Can you work these out from the model? Positions are in its coordinate system, mm. Face numbers are marked on the shaded views. A direction names the side the tool comes from. Coordinates: 2 decimals unless noted, no trailing zeros. Loops run counter-clockwise (first coordinate to the right, second up) from the corner with the lowest first, then second, coordinate; pieces in that order, holes last.
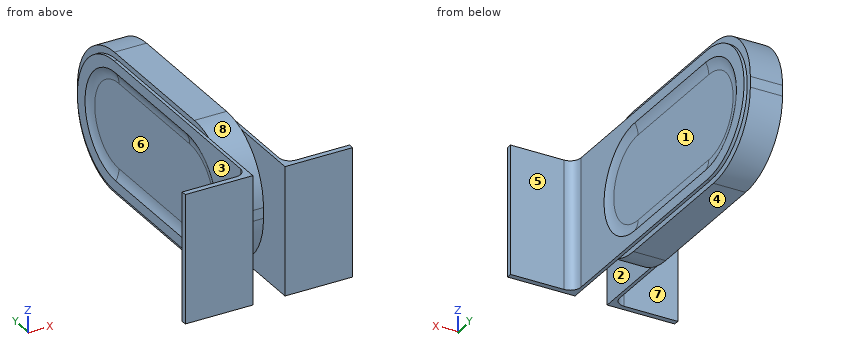
```python
from build123d import *

# Parameters (mm, degrees)
BOSS_EXTRUDE1_DEPTH = 15
BOSS_EXTRUDE2_DEPTH = 3
FILLET1_R           = 20
SKETCH4_W           = 60
SKETCH4_H           = 120
BOSS_EXTRUDE3_DEPTH = 5
BOSS_EXTRUDE4_START = -30
BOSS_EXTRUDE4_DEPTH = 3
FILLET2_R           = 20
FILLET4_R           = 10
BOSS_EXTRUDE5_START = -5
BOSS_EXTRUDE5_DEPTH = 120


with BuildPart() as part:
    # Sketch1 → Boss-Extrude1 (new, symmetric)
    with BuildSketch(Plane(origin=(0, 0, 0), x_dir=(0, 0, -1), z_dir=(1, 0, 0))):
        with BuildLine():
            Line((5, 125), (-5, 125))
            ThreePointArc((-5, 125), (-47.426406871, 107.426406871), (-65, 65))
            Line((-65, 65), (-65, -65))
            ThreePointArc((-65, -65), (-47.426406871, -107.426406871), (-5, -125))
            Line((-5, -125), (5, -125))
            ThreePointArc((5, -125), (47.426406871, -107.426406871), (65, -65))
            Line((65, -65), (65, 65))
            ThreePointArc((65, 65), (47.426406871, 107.426406871), (5, 125))
        make_face()
    extrude(amount=BOSS_EXTRUDE1_DEPTH, both=True)

    # Sketch3 → Boss-Extrude2 (add)
    with BuildSketch(Plane(origin=(15, 0, 0), x_dir=(0, 0, -1), z_dir=(1, 0, 0))):
        with BuildLine():
            Line((-60, -60), (-60, 60))
            ThreePointArc((-60, 60), (0, 120), (60, 60))
            Line((60, 60), (60, -60))
            Line((60, -60), (60, -160))
            Line((60, -160), (-60, -160))
            Line((-60, -160), (-60, -60))
        make_face()
        with BuildLine():
            Line((-50, -57.5), (-50, 57.5))
            ThreePointArc((-50, 57.5), (0, 107.5), (50, 57.5))
            Line((50, 57.5), (50, -57.5))
            ThreePointArc((50, -57.5), (0, -107.5), (-50, -57.5))
        make_face(mode=Mode.SUBTRACT)
    extrude(amount=BOSS_EXTRUDE2_DEPTH)

    # Fillet1
    # the kernel refuses this fillet: 20 mm, written as the material it adds along each edge
    with BuildSketch(Plane(origin=(15, 57.5, -50), x_dir=(1, 0, 0), z_dir=(0, -1, 0)), Plane(origin=(15, -57.5, 50), x_dir=(1, 0, 0), z_dir=(0, 1, 0))) as fillet1_piece_1:
        with BuildLine():
            CenterArc((20, 10.535653753), FILLET1_R, 180, 31.788330617)
            Line((0, 10.535653753), (-0.4, 10.535653753))
            Line((-0.4, 10.535653753), (-0.4, 0))
            Line((-0.4, 0), (0, -0.4))
            ThreePointArc((0, -0.4), (1.5, -0.4), (2.66, -0.210713075))
            Line((2.66, -0.210713075), (3, 0))
        make_face()
    extrude(amount=115)
    with BuildSketch(Plane(origin=(15, -57.5, 0), x_dir=(0, 0, -1), z_dir=(0, 1, 0))) as fillet1_piece_2:
        with BuildLine():
            CenterArc((39.464346247, -20), FILLET1_R, 58.211669383, 31.788330617)
            Line((39.464346247, 0), (39.464346247, 0.4))
            Line((39.464346247, 0.4), (50, 0.4))
            Line((50, 0.4), (50.4, 0))
            ThreePointArc((50.4, 0), (50.4, -1.5), (50.210713075, -2.66))
            Line((50.210713075, -2.66), (50, -3))
        make_face()
    revolve(axis=Axis((15, -57.5, 0), (-1, 0, 0)), revolution_arc=180)
    with BuildSketch(Plane(origin=(15, 57.5, 0), x_dir=(0, 0, 1), z_dir=(0, -1, 0))) as fillet1_piece_3:
        with BuildLine():
            CenterArc((39.464346247, -20), FILLET1_R, 58.211669383, 31.788330617)
            Line((39.464346247, 0), (39.464346247, 0.4))
            Line((39.464346247, 0.4), (50, 0.4))
            Line((50, 0.4), (50.4, 0))
            ThreePointArc((50.4, 0), (50.4, -1.5), (50.210713075, -2.66))
            Line((50.210713075, -2.66), (50, -3))
        make_face()
    revolve(axis=Axis((15, 57.5, 0), (-1, 0, 0)), revolution_arc=180)

    # Sketch4 → Boss-Extrude3 (add)
    with BuildSketch(Plane.XZ.offset(160)):
        with Locations((48, 0)):
            Rectangle(SKETCH4_W, SKETCH4_H)
        with Locations((-48, 0)):
            Rectangle(SKETCH4_W, SKETCH4_H)
    extrude(amount=-BOSS_EXTRUDE3_DEPTH)


with BuildPart() as boss_extrude3_piece_1:
    # of the separate pieces the step leaves, piece 1, a body of its own (boss_extrude3_pieces)
    add(part.part.solids().sort_by_distance((18, 57.5, 50))[0])

    # Sketch3<4> → Boss-Extrude4 (add)
    with BuildSketch(Plane(origin=(15, 0, 0), x_dir=(0, 0, -1), z_dir=(1, 0, 0)).offset(BOSS_EXTRUDE4_START)):
        with BuildLine():
            Line((-60, -60), (-60, 60))
            ThreePointArc((-60, 60), (0, 120), (60, 60))
            Line((60, 60), (60, -60))
            Line((60, -60), (60, -160))
            Line((60, -160), (-60, -160))
            Line((-60, -160), (-60, -60))
        make_face()
        with BuildLine():
            Line((-50, -57.5), (-50, 57.5))
            ThreePointArc((-50, 57.5), (0, 107.5), (50, 57.5))
            Line((50, 57.5), (50, -57.5))
            ThreePointArc((50, -57.5), (0, -107.5), (-50, -57.5))
        make_face(mode=Mode.SUBTRACT)
    extrude(amount=-BOSS_EXTRUDE4_DEPTH)

    # Fillet2
    # the kernel refuses this fillet: 20 mm, written as the material it adds along each edge
    with BuildSketch(Plane(origin=(-15, -57.5, 0), x_dir=(0, 0, -1), z_dir=(0, 1, 0))) as fillet2_piece_1:
        with BuildLine():
            CenterArc((39.464346247, 20), FILLET2_R, 270, 31.788330617)
            Line((39.464346247, 0), (39.464346247, -0.4))
            Line((39.464346247, -0.4), (50, -0.4))
            Line((50, -0.4), (50.4, 0))
            ThreePointArc((50.4, 0), (50.4, 1.5), (50.210713075, 2.66))
            Line((50.210713075, 2.66), (50, 3))
        make_face()
    revolve(axis=Axis((-15, -57.5, 0), (-1, 0, 0)), revolution_arc=180)
    with BuildSketch(Plane(origin=(-15, -57.5, 50), x_dir=(-1, 0, 0), z_dir=(0, 1, 0)), Plane(origin=(-15, 57.5, -50), x_dir=(-1, 0, 0), z_dir=(0, -1, 0))) as fillet2_piece_2:
        with BuildLine():
            CenterArc((20, -10.535653753), FILLET2_R, 148.211669383, 31.788330617)
            Line((0, -10.535653753), (-0.4, -10.535653753))
            Line((-0.4, -10.535653753), (-0.4, 0))
            Line((-0.4, 0), (0, 0.4))
            ThreePointArc((0, 0.4), (1.5, 0.4), (2.66, 0.210713075))
            Line((2.66, 0.210713075), (3, 0))
        make_face()
    extrude(amount=115)
    with BuildSketch(Plane(origin=(-15, 57.5, 0), x_dir=(0, 0, 1), z_dir=(0, -1, 0))) as fillet2_piece_3:
        with BuildLine():
            CenterArc((39.464346247, 20), FILLET2_R, 270, 31.788330617)
            Line((39.464346247, 0), (39.464346247, -0.4))
            Line((39.464346247, -0.4), (50, -0.4))
            Line((50, -0.4), (50.4, 0))
            ThreePointArc((50.4, 0), (50.4, 1.5), (50.210713075, 2.66))
            Line((50.210713075, 2.66), (50, 3))
        make_face()
    revolve(axis=Axis((-15, 57.5, 0), (-1, 0, 0)), revolution_arc=180)

    # Fillet4
    fillet4_edges = [boss_extrude3_piece_1.edges().sort_by_distance(p)[0] for p in [
        (18, -155, 0),
    ]]
    fillet(fillet4_edges, radius=FILLET4_R)



with BuildPart() as boss_extrude3_piece_2:
    # of the separate pieces the step leaves, piece 2, a body of its own (boss_extrude3_pieces)
    add(part.part.solids().sort_by_distance((-18, -160, 60))[0])


with BuildPart() as boss_extrude3_piece_1_1:
    add(boss_extrude3_piece_1.part)

    add(boss_extrude3_piece_2.part)  # Boss-Extrude5 merges Boss-Extrude3 piece 2
    # Sketch5 → Boss-Extrude5 (add)
    with BuildSketch(Plane.XY.offset(65).offset(BOSS_EXTRUDE5_START)):
        with BuildLine():
            Line((-28, -155), (-18, -155))
            Line((-18, -155), (-18, -145))
            ThreePointArc((-18, -145), (-20.928932188, -152.071067812), (-28, -155))
        make_face()
    extrude(amount=-BOSS_EXTRUDE5_DEPTH)


solid = boss_extrude3_piece_1_1.part
```
(1) I'm going to push flat-ended pins straight in: pin 1 (4 mm diameter, centred on x = -14.5, y = -104.5, fed in from +Z); pin 2 (5 mm diameter, centred on x = 40, z = -45, fed in from +Y); pin 3 (5 mm diameter, centred on y = 59, z = 3.5, fed in from -X). Where does each tip first touch, or does it pass through?
Check values:
pin 1: stops at z = 60
pin 2: stops at y = -155
pin 3: stops at x = -15
(2) If we mould it in two halves opening along Y, with no side actions, what happens to the marked faces 6, 7 and 8? For each: released by +Y, released by -Y, zero draft, split by the parting line, or undercut.
Check values:
face 6: undercut
face 7: released by +Y
face 8: released by -Y
(3) I want a section at D-D on x = 48.5. Write out the boundary of the cut face in (y, z).
Check values:
outline: (-160, -60) - (-155, -60) - (-155, 60) - (-160, 60) - close
(4) I want a section at B-B on z = 0. Write out the boundary of the cut face in (x, y).
Check values:
outline: (-78, -160) - (-15, -160) - (-15, -125) - (15, -125) - (15, -160) - (78, -160) - (78, -155) - (28, -155) arc R10 cw to (18, -145) - (18, -107.5) arc R20 cw to (15, -96.96) - (15, 96.96) arc R20 cw to (18, 107.5) - (18, 120) - (15, 120) - (15, 125) - (-15, 125) - (-15, 120) - (-18, 120) - (-18, 107.5) arc R20 cw to (-15, 96.96) - (-15, -96.96) arc R20 cw to (-18, -107.5) - (-18, -145) arc R10 cw to (-28, -155) - (-78, -155) - close
(5) If I drill on probe 1 along X at (y, z) = (-128, 9); probe 2 along Y at (x, z) = (-30, -21.5); probe 3 along X at (y, z) = (-115, 14), over which ranges is the centre line in solid material (lowest first)?
Check values:
probe 1: x = -18 to -15, 15 to 18
probe 2: y = -160 to -155
probe 3: x = -18 to 18
(6) Which directions (+Z, -Z, +X, -X, +Y, -Y) give clear straight access to the entire face, cutting with the end or side of a thin tool? Please do the marked faces 1, 2, 3, 4 and 5.
Check values:
face 1: +X
face 2: -Y
face 3: +Z, -Z, -X, +Y
face 4: -Z, +X, -X, +Y, -Y
face 5: +Z, -Z, +X, +Y
(7) I want a section at A-A on y = -25. Write out the boundary of the cut face in (x, z), then the cut area to 3 significant figures.
Check values:
outline: (-18, -60) - (-15, -60) - (-15, -65) - (15, -65) - (15, -60) - (18, -60) - (18, -50) arc R20 cw to (15, -39.46) - (15, 39.46) arc R20 cw to (18, 50) - (18, 60) - (15, 60) - (15, 65) - (-15, 65) - (-15, 60) - (-18, 60) - (-18, 50) arc R20 cw to (-15, 39.46) - (-15, -39.46) arc R20 cw to (-18, -50) - close
area: 4,060 mm2
(8) I want a section at C-C on x = 7. Write out the boundary of the cut face in (y, z).
Check values:
outline: (-125, -5) arc R60 ccw to (-65, -65) - (65, -65) arc R60 ccw to (125, -5) - (125, 5) arc R60 ccw to (65, 65) - (-65, 65) arc R60 ccw to (-125, 5) - close
